Source: CAD feature listing. Evaluate the final solid. Frame: model axes, mm. A direction names the side the tool comes from. Round coordinates to 2 decimals unless told otherwise and drop trailing zeros. Write each loop counter-clockwise with the first axis right and the second up, starting at its lowest first coordinate (ties: lowest second). Pieces come first, ordered by that corner, then holes. Notation, with made-up numbers: M 88,10.5 L 96,10.5 A20 cw 96,30.5 Z; hole C -5.75,-21 d8. An arc over 180 degrees is marked long. Put each result on its own line as item: value. Start each with the question number.
```python
from build123d import *

# Parameters (mm, degrees)
F1_DEPTH = 6.35
F2_W     = 38.1
F2_H     = 68.58
F3_DEPTH = 19.05
F4_T     = -2.54
F6_DEPTH = 19.05
F7_T     = -2.54
F9_DEPTH = 19.05


# Not quite as in the source:
# - a shell that OpenCascade refuses in one call is made with other operations: the cavity is built on its own and cut out


with BuildPart() as f1:
    # F0 (on Front) → F1 (new body)
    with BuildSketch(Plane.XZ):
        Polygon((-90.1848339975, 87.6345549519), (-90.1848339975, -90.1654450481), (87.6151660025, -90.1654450481), (87.6151660025, 87.6345549519), (11.4151660025, 87.6345549519), (11.4151660025, 36.8345549519), (-13.9848339975, 36.8345549519), (-13.9848339975, 87.6345549519), align=None)
    extrude(amount=F1_DEPTH)

    # F2 (on Front) → F3 (join)
    with BuildSketch(Plane.XZ):
        with Locations((-53.5051479423, 45.5094583845)):
            Rectangle(F2_W, F2_H)
    extrude(amount=F3_DEPTH)

    # F4
    f4_openings = [f1.faces().sort_by_distance(p)[0] for p in [
        (-53.505148, -19.05, 45.509458),
    ]]
    offset(amount=F4_T, openings=f4_openings, kind=Kind.INTERSECTION)

    # F5 (on Front) → F6 (join)
    with BuildSketch(Plane.XZ):
        Polygon((12.6932561398, 77.6492066986), (12.6932561398, 8.7867740487), (66.0325084011, 9.0692066986), (66.0325084011, 77.6492066986), align=None)
    extrude(amount=F6_DEPTH)

    # F7: a shell. OpenCascade refuses it in one call, so the cavity is built on its own and cut out:
    # the body offset inwards by the wall thickness, plus a prism from it out through each open face.
    f7_core = offset(f1.part, amount=F7_T, kind=Kind.INTERSECTION, mode=Mode.PRIVATE)
    f7_exits = [f7_core.faces().sort_by_distance(p)[0] for p in [
        (39.346735, -16.51, 43.288574),
    ]]
    add(f7_core, mode=Mode.SUBTRACT)
    extrude(f7_exits, amount=-F7_T, mode=Mode.SUBTRACT)

    # F8 (on Front) → F9 (join)
    with BuildSketch(Plane.XZ):
        Polygon((38.4033048588, 0), (-37.7966951412, 0), (-37.7966951412, -38.1), (-32.7166951412, -38.1), (-32.7166951412, -5.08), (33.3233048588, -5.08), (33.3233048588, -38.1), (38.4033048588, -38.1), align=None)
    extrude(amount=F9_DEPTH)


solid = f1.part
```
(1) Pull-direction query (Z, two-part tool) for faces 6 (the flat face through (66.033, -13, 43)), 7 (the flat face through (-2, -2.54, -19)), 8 (the flat face through (-1, -3, 36.835)), 9 (the flat face through (-2, -3.81, -19)); classes: +Z half, -Z half, draft (parallel to the pull), parting line (faces both ways), or undercut.
(2) Section query A-A (z = 57). Count the separate pieces of the cut face and the enclosed holes in it, and give its area (3 significant figures).
(3) Section query B-B (y = -14). Return loops of the section in (x, z).
(4) Ray query, line 1 along X through (y, z) = (-14.5, 61); line 2 along Z through (x, y) = (-6, -3); line 3 along X through (y, z) = (-5.75, 34.5). Return the intervals inside material, ascending.
(5) Contact query for flat-ended pins moving along their axis: P1, Ø3, axis at y = -15.5, z = 17, coming from the +X side; P2, Ø6.5, axis at x = 40, y = -14.5, coming from the +Z side; P3, Ø6.5, axis at x = -62, y = -12, coming from the +Z side. Output: stop coordinate, or through.
(6) Section query C-C (x = -4.5). Return loops of the section in (y, z).
(7) Access query for faces 1 (the flat face through (-13.985, -3, 62)), 2 (the flat face through (-32.717, -13, -22)), 3 (the flat face through (-37.797, -13, -19)), 4 (the flat face through (-70.015, -11, 45)), 5 (the flat face through (-72.555, -13, 45)). Directions: +Z, -Z, +X, -X, +Y, -Y. A direction counts if a zero-diameter tool reaches every point of the face in a straight line with its end or side. Return the directions, or none.
(8) Section query D-D (z = 32). Return loops of the section in (x, y).
Entries:
1. face 6: draft
1. face 7: undercut
1. face 8: +Z half
1. face 9: undercut
2. separate pieces: 2
2. enclosed holes: 1
2. area: 713 mm2
3. outline: M -72.56,11.22 L -34.46,11.22 L -34.46,79.8 L -72.56,79.8 Z; M -37.8,-38.1 L -32.72,-38.1 L -32.72,-5.08 L 33.32,-5.08 L 33.32,-38.1 L 38.4,-38.1 L 38.4,0 L -37.8,0 Z; M 12.69,8.79 L 66.03,9.07 L 66.03,77.65 L 12.69,77.65 Z; hole M -70.02,13.76 L -37,13.76 L -37,77.26 L -70.02,77.26 Z; hole M 15.23,11.34 L 63.49,11.6 L 63.49,75.11 L 15.23,75.11 Z
4. line 1: -72.56 to -70.02, -37 to -34.46, 12.69 to 15.23, 63.49 to 66.03
4. line 2: -90.17 to -87.63, -5.08 to 0, 34.29 to 36.83
4. line 3: -90.18 to -70.02, -37 to 15.23, 63.49 to 87.62
5. P1: x = 66.03
5. P2: z = 77.65
5. P3: z = 79.8
6. outline: M -19.05,-5.08 L -6.35,-5.08 L -6.35,-90.17 L 0,-90.17 L 0,36.83 L -6.35,36.83 L -6.35,0 L -19.05,0 Z; hole M -3.81,-87.63 L -2.54,-87.63 L -2.54,-5.08 L -3.81,-5.08 Z; hole M -3.81,0 L -2.54,0 L -2.54,34.29 L -3.81,34.29 Z
7. face 1: +Z, +Y, -Y
7. face 2: -Z, -Y
7. face 3: -Z, -X, -Y
7. face 4: -Y
7. face 5: +Z, -Z, -X, -Y
8. outline: M -90.18,-6.35 L -72.56,-6.35 L -72.56,-19.05 L -70.02,-19.05 L -70.02,-3.81 L -87.64,-3.81 L -87.64,-2.54 L 12.69,-2.54 L 12.69,-3.81 L -37,-3.81 L -37,-19.05 L -34.46,-19.05 L -34.46,-6.35 L 12.69,-6.35 L 12.69,-19.05 L 15.23,-19.05 L 15.23,-2.54 L 63.49,-2.54 L 63.49,-19.05 L 66.03,-19.05 L 66.03,-6.35 L 87.62,-6.35 L 87.62,0 L -90.18,0 Z; hole M 66.03,-3.81 L 85.08,-3.81 L 85.08,-2.54 L 66.03,-2.54 Z
